Read the model definition and answer for the solid it produces. Units are mm, in the model's axes. A direction names the side the tool comes from. Coordinates: 2 decimals unless noted, no trailing zeros. Order: outer loops, then holes, each group sorted by start corner. A loop starts at its lowest first (then second) coordinate and runs counter-clockwise, first axis right, second up. Notation, with made-up numbers: (11.25, 2.25) - (15.25, 2.25) arc R24 cw to (15.25, 23.25) - close; hole circle Ø3 at (74.25, 9). An arc over 180 degrees is marked (long way). Use one line per item in the form item = value.
```python
from build123d import *

# Parameters (mm, degrees)
SKETCH1_W           = 60
SKETCH1_H           = 60
BOSS_EXTRUDE1_DEPTH = 10
FILLET1_R           = 2
FILLET2_R           = 2
SKETCH3_R           = 15
SKETCH3_R_2         = 13
BOSS_EXTRUDE2_DEPTH = 20
CUT_EXTRUDE1_START  = -20
SKETCH4_R           = 13
CUT_EXTRUDE1_DEPTH  = 20
BOSS_EXTRUDE4_START = -20
BOSS_EXTRUDE4_DEPTH = 20
FILLET5_R           = 2
CUT_EXTRUDE2_REACH  = 83.874
SKETCH12_R          = 2.25
SKETCH13_R          = 5
CUT_EXTRUDE3_DEPTH  = 12
CUT_EXTRUDE4_START  = 12
SKETCH14_R          = 5
CUT_EXTRUDE4_DEPTH  = 12
CUT_EXTRUDE12_START = -20
CUT_EXTRUDE12_DEPTH = 20


with BuildPart() as part:
    # Sketch1 → Boss-Extrude1 (new body)
    with BuildSketch(Plane.XY):
        Rectangle(SKETCH1_W, SKETCH1_H)
    extrude(amount=BOSS_EXTRUDE1_DEPTH)

    # Sketch2 → Revolve1 (revolve)
    with BuildSketch(Plane(origin=(0, 0, 0), x_dir=(1, 0, 0), z_dir=(0, 1, 0)), mode=Mode.PRIVATE) as revolve1_sk:
        Polygon((-25, -10), (-15, -37.474774195), (0, -37.474774195), (0, -10), align=None)
    revolve(revolve1_sk.sketch.rotate(Axis((0, 0, 38.640996606), (0, 0, -1)), 180), axis=Axis((0, 0, 38.640996606), (0, 0, -1)))

    # Fillet1
    fillet1_edges = [part.edges().sort_by_distance(p)[0] for p in [
        (30, 0, 10),
        (0, 30, 10),
        (-25, 0, 10),
        (-30, 0, 10),
        (0, -30, 10),
    ]]
    fillet(fillet1_edges, radius=FILLET1_R)

    # Fillet2
    # the kernel refuses this fillet: 2 mm, written as the material it takes off along each edge
    with BuildSketch(Plane(origin=(28, -28, 8), x_dir=(0, -1, 0), z_dir=(1, 0, 0))) as fillet2_piece_1_section:
        Polygon((0, 0), (FILLET2_R, 0), (FILLET2_R, -FILLET2_R), (0, -FILLET2_R), align=None)
    fillet2_piece_1 = extrude(amount=FILLET2_R, mode=Mode.PRIVATE)
    fillet2_piece_1 = fillet2_piece_1 - Plane(origin=(28, -28, 8), x_dir=(0, 0.7071067811865475, -0.7071067811865475), z_dir=(1, 0, 0)) * Sphere(FILLET2_R, mode=Mode.PRIVATE)
    add(fillet2_piece_1, mode=Mode.SUBTRACT)
    with BuildSketch(Plane(origin=(-28, -28, 8), x_dir=(0, -1, 0), z_dir=(-1, 0, 0))) as fillet2_piece_2_section:
        Polygon((0, 0), (FILLET2_R, 0), (FILLET2_R, FILLET2_R), (0, FILLET2_R), align=None)
    fillet2_piece_2 = extrude(amount=FILLET2_R, mode=Mode.PRIVATE)
    fillet2_piece_2 = fillet2_piece_2 - Plane(origin=(-28, -28, 8), x_dir=(0, 0.7071067811865475, -0.7071067811865475), z_dir=(-1, 0, 0)) * Sphere(FILLET2_R, mode=Mode.PRIVATE)
    add(fillet2_piece_2, mode=Mode.SUBTRACT)
    with BuildSketch(Plane(origin=(28, 28, 8), x_dir=(1, 0, 0), z_dir=(0, 1, 0))) as fillet2_piece_3_section:
        Polygon((0, 0), (FILLET2_R, 0), (FILLET2_R, -FILLET2_R), (0, -FILLET2_R), align=None)
    fillet2_piece_3 = extrude(amount=FILLET2_R, mode=Mode.PRIVATE)
    fillet2_piece_3 = fillet2_piece_3 - Plane(origin=(28, 28, 8), x_dir=(-0.7071067811865475, 0, -0.7071067811865475), z_dir=(0, 1, 0)) * Sphere(FILLET2_R, mode=Mode.PRIVATE)
    add(fillet2_piece_3, mode=Mode.SUBTRACT)
    with BuildSketch(Plane(origin=(-28, 28, 8), x_dir=(-1, 0, 0), z_dir=(0, 1, 0))) as fillet2_piece_4_section:
        Polygon((0, 0), (FILLET2_R, 0), (FILLET2_R, FILLET2_R), (0, FILLET2_R), align=None)
    fillet2_piece_4 = extrude(amount=FILLET2_R, mode=Mode.PRIVATE)
    fillet2_piece_4 = fillet2_piece_4 - Plane(origin=(-28, 28, 8), x_dir=(0.7071067811865475, 0, -0.7071067811865475), z_dir=(0, 1, 0)) * Sphere(FILLET2_R, mode=Mode.PRIVATE)
    add(fillet2_piece_4, mode=Mode.SUBTRACT)
    with BuildSketch(Plane(origin=(-30, 30, -5), x_dir=(1, 0, 0), z_dir=(0, 0, 1)), Plane(origin=(-30, -30, -5), x_dir=(0, 1, 0), z_dir=(0, 0, 1))) as fillet2_piece_5:
        with BuildLine():
            CenterArc((FILLET2_R, -FILLET2_R), FILLET2_R, 90, 90)
            Line((0, -FILLET2_R), (0, 0))
            Line((0, 0), (FILLET2_R, 0))
        make_face()
    extrude(amount=13, mode=Mode.SUBTRACT)
    with BuildSketch(Plane(origin=(30, 30, -5), x_dir=(-1, 0, 0), z_dir=(0, 0, 1)), Plane(origin=(30, -30, -5), x_dir=(0, 1, 0), z_dir=(0, 0, 1))) as fillet2_piece_6:
        with BuildLine():
            CenterArc((FILLET2_R, FILLET2_R), FILLET2_R, 180, 90)
            Line((0, FILLET2_R), (0, 0))
            Line((0, 0), (FILLET2_R, 0))
        make_face()
    extrude(amount=13, mode=Mode.SUBTRACT)

    # Sketch3 → Boss-Extrude2 (add)
    with BuildSketch(Plane.XY.offset(37.474774195)):
        Circle(SKETCH3_R)
        Circle(SKETCH3_R_2, mode=Mode.SUBTRACT)
    extrude(amount=BOSS_EXTRUDE2_DEPTH)

    # Sketch4 → Cut-Extrude1 (cut)
    with BuildSketch(Plane.XY.offset(37.474774195).offset(CUT_EXTRUDE1_START)):
        Circle(SKETCH4_R)
    extrude(amount=CUT_EXTRUDE1_DEPTH, mode=Mode.SUBTRACT)

    # Sketch7 → Boss-Extrude4 (add)
    with BuildSketch(Plane.XY.offset(57.474774195).offset(BOSS_EXTRUDE4_START)):
        with BuildLine():
            Line((4.148885958, 14.41480993), (28.173569174, 7.5))
            Line((28.173569174, 7.5), (28.173569174, -7.5))
            Line((28.173569174, -7.5), (4.148885958, -14.41480993))
            ThreePointArc((4.148885958, -14.41480993), (15, 0), (4.148885958, 14.41480993))
        make_face()
    extrude(amount=BOSS_EXTRUDE4_DEPTH)

    # Fillet5
    fillet5_edges = [part.edges().sort_by_distance(p)[0] for p in [
        (28.173569174, 7.5, 47.474774195),
        (28.173569174, -7.5, 47.474774195),
    ]]
    fillet(fillet5_edges, radius=FILLET5_R)

    # Cut-Extrude2: up to this plane
    cut_extrude2_end = Plane(origin=(4.148885958, -14.41480993, 37.474774195), z_dir=(0.27659239718755785, -0.9609873286459298, 0))
    # Sketch12 → Cut-Extrude2 (cut, up to the surface)
    with BuildSketch(Plane(origin=(0, 20, 0), x_dir=(1, 0, 0), z_dir=(0, 1, 0)), mode=Mode.PRIVATE) as cut_extrude2_sk1:
        with Locations(Location((19.148885958, -47.474774195, 0), (0, 0, 180))):
            Circle(SKETCH12_R)
    cut_extrude2_tool1 = split(extrude(cut_extrude2_sk1.sketch, amount=-CUT_EXTRUDE2_REACH, mode=Mode.PRIVATE), bisect_by=cut_extrude2_end, keep=Keep.BOTH, mode=Mode.PRIVATE)
    add(cut_extrude2_tool1.solids().sort_by_distance((19.148886, 20, 47.474774))[0], mode=Mode.SUBTRACT)

    # Sketch13 → Cut-Extrude3 (cut)
    with BuildSketch(Plane(origin=(0, 20, 0), x_dir=(1, 0, 0), z_dir=(0, 1, 0))):
        with Locations(Location((19.148885958, -47.474774195, 0), (0, 0, 270))):
            Circle(SKETCH13_R)
    extrude(amount=-CUT_EXTRUDE3_DEPTH, mode=Mode.SUBTRACT)

    # Sketch14 → Cut-Extrude4 (cut)
    with BuildSketch(Plane(origin=(0, -20, 0), x_dir=(1, 0, 0), z_dir=(0, 1, 0)).offset(CUT_EXTRUDE4_START)):
        with Locations(Location((19.148885958, -47.474774195, 0), (0, 0, 270))):
            Circle(SKETCH14_R)
    extrude(amount=-CUT_EXTRUDE4_DEPTH, mode=Mode.SUBTRACT)

    # Sketch15 → Cut-Extrude12 (cut)
    with BuildSketch(Plane.XY.offset(57.474774195).offset(CUT_EXTRUDE12_START)):
        with BuildLine():
            Line((28.173569174, 1), (12.961481397, 1))
            ThreePointArc((12.961481397, 1), (13, 0), (12.961481397, -1))
            Line((12.961481397, -1), (28.173569174, -1))
            Line((28.173569174, -1), (28.173569174, 1))
        make_face()
    extrude(amount=CUT_EXTRUDE12_DEPTH, mode=Mode.SUBTRACT)


solid = part.part
```
(1) Straight lines are drawn through the part: L1, parallel to X at y = -3, z = 48; L2, parallel to Z at x = 8.5, y = 3; L3, parallel to X at y = -8, z = 24. For each, find the intervals that lie inside material, in ascending order.
Answer list:
L1 = -14.7 to -12.65, 12.65 to 16.96, 21.34 to 28.17
L2 = 0 to 17.47
L3 = -18.23 to -10.25, 10.25 to 18.23
(2) Section A-A, the plane z = 54.5 is taken. Write down the section's boundary in (x, y).
Answer list:
outline = (4.15, -14.41) - (26.73, -7.92) arc R2 ccw to (28.17, -5.99) - (28.17, -1) - (12.96, -1) arc R13 cw (long way) to (12.96, 1) - (28.17, 1) - (28.17, 5.99) arc R2 ccw to (26.73, 7.92) - (4.15, 14.41) arc R15 ccw (long way) to start
(3) Section D-D, the plane z = 29 is taken. Write down the section's boundary in (x, y), then the cut area to 3 significant figures.
Answer list:
outline = circle Ø36.17 at (0, 0); hole circle Ø26 at (0, 0)
area = 497 mm2
(4) Which of the six approach directions +Z, -Z, +X, -X, +Y, -Y give full straight-line access (tool end or side, diameter ignored) to faces 4 (the flat face through (0, 0, 17.475)), 5 (the flat face through (22, -1, 47)), 6 (the conical face through (17, -5, 30)), 7 (the flat face through (28.174, -3, 47))?
Answer list:
face_4 = +Z
face_5 = +Z, +X
face_6 = none
face_7 = +Z, +X, +Y, -Y
(5) Given pin 1 Ø23.5 at (x, y) = (0, 0) entering from +Z; pin 2 Ø1.5 at (x, z) = (8.5, 39) entering from +Y; pin 3 Ø3 at (x, z) = (20.5, 47) entering from -Y, each flat-ended and moving along its own axis, determine where each tip first touches the part or whether it passes through.
Answer list:
pin_1 = 17.47
pin_2 = 13.38
pin_3 = -8
(6) Section C-C, the plane y = 0 is taken. Write down the section's boundary in (x, z), then the cut area to 3 significant figures.
Answer list:
outline = (-30, 0) - (30, 0) - (30, 8) arc R2 ccw to (28, 10) - (26.4, 10) arc R2 cw to (24.52, 11.32) - (15, 37.47) - (13, 37.47) - (13, 17.47) - (-13, 17.47) - (-13, 57.47) - (-15, 57.47) - (-15, 37.47) - (-24.52, 11.32) arc R2 cw to (-26.4, 10) - (-28, 10) arc R2 ccw to (-30, 8) - close
area = 1,220 mm2
(7) Section B-B, the plane x = 0 is taken. Write down the section's boundary in (y, z), then the cut area to 3 significant figures.
Answer list:
outline = (-30, 0) - (30, 0) - (30, 8) arc R2 ccw to (28, 10) - (26.4, 10) arc R2 cw to (24.52, 11.32) - (15, 37.47) - (15, 57.47) - (13, 57.47) - (13, 17.47) - (-13, 17.47) - (-13, 57.47) - (-15, 57.47) - (-15, 37.47) - (-24.52, 11.32) arc R2 cw to (-26.4, 10) - (-28, 10) arc R2 ccw to (-30, 8) - close
area = 1,260 mm2
(8) The mould has two halves that part along X. Classify faces 1 (the cylindrical face through (12.4, 3.9, 37.2)), 2 (the flat face through (22, 1, 47)), 3 (the flat face through (-30, 0, 4)): +X half, -X half, draft (parallel to the pull), parting line (faces both ways), or undercut.
Answer list:
face_1 = undercut
face_2 = draft
face_3 = -X half
